from build123d import *

# Parameters (mm, degrees)
RECTANGLE130_AS_DRAWN_W                      = 25
RECTANGLE130_AS_DRAWN_H                      = 3
EXTRUDE152_DEPTH                             = 3
EXTRUDE152_ONTO_RECTANGLE130_ROLL_ANGLE      = -90
EXTRUDE152_ONTO_RECTANGLE130_PLACEMENT_ANGLE = 180
RECTANGLE128_AS_DRAWN_W                      = 25
RECTANGLE128_AS_DRAWN_H                      = 3
EXTRUDE153_DEPTH                             = 3
EXTRUDE153_ONTO_RECTANGLE128_ROLL_ANGLE      = -90
EXTRUDE153_ONTO_RECTANGLE128_PLACEMENT_ANGLE = 180
RECTANGLE132_AS_DRAWN_W                      = 3
RECTANGLE132_AS_DRAWN_H                      = 19.5
EXTRUDE166_DEPTH                             = 3
EXTRUDE166_ONTO_RECTANGLE132_ROLL_ANGLE      = -90
EXTRUDE166_ONTO_RECTANGLE132_PLACEMENT_ANGLE = 180
RECTANGLE127_AS_DRAWN_W                      = 25
RECTANGLE127_AS_DRAWN_H                      = 3
EXTRUDE147_DEPTH                             = 3
EXTRUDE147_ONTO_RECTANGLE127_ROLL_ANGLE      = -90
EXTRUDE147_ONTO_RECTANGLE127_PLACEMENT_ANGLE = 180
RECTANGLE129_AS_DRAWN_W                      = 25
RECTANGLE129_AS_DRAWN_H                      = 3
EXTRUDE149_DEPTH                             = 3
EXTRUDE149_ONTO_RECTANGLE129_ROLL_ANGLE      = -90
EXTRUDE149_ONTO_RECTANGLE129_PLACEMENT_ANGLE = 180
BOX045_W                                     = 100
BOX045_H                                     = 3
BOX045_DEPTH                                 = 45


with BuildPart() as extrude152:
    # Rectangle130 as drawn → Extrude152 (new)
    with BuildSketch(Plane.XY):
        with Locations((12.5, 1.5)):
            Rectangle(RECTANGLE130_AS_DRAWN_W, RECTANGLE130_AS_DRAWN_H)
    extrude(amount=-EXTRUDE152_DEPTH)


with BuildPart() as extrude152_1:
    # Extrude152 onto Rectangle130 roll: moved
    add(extrude152.part.rotate(Axis((0, 0, 0), (1, 0, 0)), EXTRUDE152_ONTO_RECTANGLE130_ROLL_ANGLE))


with BuildPart() as extrude152_2:
    # Extrude152 onto Rectangle130 placement: moved
    add(extrude152_1.part.moved(Location((39, -77, -70))).rotate(Axis((39, -77, -70), (0, 0, 1)), EXTRUDE152_ONTO_RECTANGLE130_PLACEMENT_ANGLE))


with BuildPart() as extrude152_3:
    # Extrude152 placement: moved
    add(extrude152_2.part.moved(Location((0, 0, -42))))


with BuildPart() as extrude153:
    # Rectangle128 as drawn → Extrude153 (new)
    with BuildSketch(Plane.XY):
        with Locations((12.5, 1.5)):
            Rectangle(RECTANGLE128_AS_DRAWN_W, RECTANGLE128_AS_DRAWN_H)
    extrude(amount=-EXTRUDE153_DEPTH)


with BuildPart() as extrude153_1:
    # Extrude153 onto Rectangle128 roll: moved
    add(extrude153.part.rotate(Axis((0, 0, 0), (1, 0, 0)), EXTRUDE153_ONTO_RECTANGLE128_ROLL_ANGLE))


with BuildPart() as extrude153_2:
    # Extrude153 onto Rectangle128 placement: moved
    add(extrude153_1.part.moved(Location((89, -77, -70))).rotate(Axis((89, -77, -70), (0, 0, 1)), EXTRUDE153_ONTO_RECTANGLE128_PLACEMENT_ANGLE))


with BuildPart() as extrude153_3:
    # Extrude153 placement: moved
    add(extrude153_2.part.moved(Location((0, 0, -42))))


with BuildPart() as extrude166:
    # Rectangle132 as drawn → Extrude166 (new)
    with BuildSketch(Plane.XY):
        with Locations((1.5, 9.75)):
            Rectangle(RECTANGLE132_AS_DRAWN_W, RECTANGLE132_AS_DRAWN_H)
    extrude(amount=-EXTRUDE166_DEPTH)


with BuildPart() as extrude166_1:
    # Extrude166 onto Rectangle132 roll: moved
    add(extrude166.part.rotate(Axis((0, 0, 0), (1, 0, 0)), EXTRUDE166_ONTO_RECTANGLE132_ROLL_ANGLE))


with BuildPart() as extrude166_2:
    # Extrude166 onto Rectangle132 placement: moved
    add(extrude166_1.part.moved(Location((114, -77, -92.5))).rotate(Axis((114, -77, -92.5), (0, 0, 1)), EXTRUDE166_ONTO_RECTANGLE132_PLACEMENT_ANGLE))


with BuildPart() as extrude147:
    # Rectangle127 as drawn → Extrude147 (new)
    with BuildSketch(Plane.XY):
        with Locations((12.5, 1.5)):
            Rectangle(RECTANGLE127_AS_DRAWN_W, RECTANGLE127_AS_DRAWN_H)
    extrude(amount=-EXTRUDE147_DEPTH)


with BuildPart() as extrude147_1:
    # Extrude147 onto Rectangle127 roll: moved
    add(extrude147.part.rotate(Axis((0, 0, 0), (1, 0, 0)), EXTRUDE147_ONTO_RECTANGLE127_ROLL_ANGLE))


with BuildPart() as extrude147_2:
    # Extrude147 onto Rectangle127 placement: moved
    add(extrude147_1.part.moved(Location((114, -77, -70))).rotate(Axis((114, -77, -70), (0, 0, 1)), EXTRUDE147_ONTO_RECTANGLE127_PLACEMENT_ANGLE))


with BuildPart() as fusion064026:
    # Rectangle129 as drawn → Extrude149 (new)
    with BuildSketch(Plane.XY):
        with Locations((12.5, 1.5)):
            Rectangle(RECTANGLE129_AS_DRAWN_W, RECTANGLE129_AS_DRAWN_H)
    extrude(amount=-EXTRUDE149_DEPTH)


with BuildPart() as fusion064026_1:
    # Extrude149 onto Rectangle129 roll: moved
    add(fusion064026.part.rotate(Axis((0, 0, 0), (1, 0, 0)), EXTRUDE149_ONTO_RECTANGLE129_ROLL_ANGLE))


with BuildPart() as fusion064026_2:
    # Extrude149 onto Rectangle129 placement: moved
    add(fusion064026_1.part.moved(Location((64, -77, -70))).rotate(Axis((64, -77, -70), (0, 0, 1)), EXTRUDE149_ONTO_RECTANGLE129_PLACEMENT_ANGLE))

    # Fusion064026: union Extrude152, Extrude153, Extrude166, Extrude147
    add(extrude152_3.part)
    add(extrude153_3.part)
    add(extrude166_2.part)
    add(extrude147_2.part)


with BuildPart() as fusion064026_3:
    # Fusion064026 placement: moved
    add(fusion064026_2.part.moved(Location((0, 152, 0))))


with BuildPart() as cut035015:
    # Box045 → Box045 (new body)
    with BuildSketch(Plane(origin=(14, 75, -115), x_dir=(1, 0, 0), z_dir=(0, 0, 1))):
        with Locations((50, 1.5)):
            Rectangle(BOX045_W, BOX045_H)
    extrude(amount=BOX045_DEPTH)

    # Cut035015: cut Fusion064026
    add(fusion064026_3.part, mode=Mode.SUBTRACT)


solid = cut035015.part
Geometry check sheet. Reference: the model listing, model coordinates, mm. A direction names the side the tool comes from. Give positions to 0.01 mm unless a question says otherwise; leave off trailing zeros. Order: outer loops, then holes, each group sorted by start corner. A loop starts at its lowest first (then second) coordinate and runs counter-clockwise, first axis right, second up. Notation, with made-up numbers: M 46.5,68 L 61.5,68 A22 cw 61.5,93 Z; hole C 87.25,44 d8. An arc over 180 degrees is marked long. Use a Markdown table: item, result.
Item 1: Section check C-C (z = -96). Record the cut outline in (x, y), and give its area (3 significant figures).
Answers follow:
| item | result |
|---|---|
| outline | M 14,75 L 111,75 L 111,78 L 14,78 Z |
| area | 291 mm2 |
Item 2: Depth check by flat-ended pin: P1, Ø1.5, axis at x = 49, y = 76.5, coming from the +Z side; P2, Ø1.5, axis at y = 77, z = -114, coming from the -X side; P3, Ø0.9, axis at y = 77, z = -100.5, coming from the +X side. Enter the tip coordinate at first touch or a pass-through.
Answers follow:
| item | result |
|---|---|
| P1 | stops at z = -73 |
| P2 | stops at x = 39 |
| P3 | stops at x = 111 |
Item 3: Material ranges on line 1 along X through (y, z) = (76.1, -112.5); line 2 along Z through (x, y) = (92, 76.4); line 3 along X through (y, z) = (75.8, -103), recorded low to high.
Answers follow:
| item | result |
|---|---|
| line 1 | x = 39 to 64, 89 to 114 |
| line 2 | z = -115 to -73 |
| line 3 | x = 14 to 111 |
Item 4: Tool access check on faces 5 (the flat face through (113, 76, -112)), 6 (the flat face through (39, 76, -113)), 7 (the flat face through (39, 76, -71)). Record the directions out of +Z, -Z, +X, -X, +Y, -Y that give a thin tool (end or side, any length) a straight path to the whole face; none if there is none.
Answers follow:
| item | result |
|---|---|
| face 5 | +X, +Y, -Y |
| face 6 | -Z, -X, +Y, -Y |
| face 7 | +Z, +Y, -Y |
Item 5: Draft check along X on faces 1 (the flat face through (14, 76, -91)), 2 (the flat face through (64, 76, -113)), 3 (the flat face through (89, 76, -113)), 4 (the flat face through (63, 75, -93)). Enter one of: +X half, -X half, draft (parallel to the pull), parting line (faces both ways), or undercut.
Answers follow:
| item | result |
|---|---|
| face 1 | -X half |
| face 2 | undercut |
| face 3 | undercut |
| face 4 | draft |
Item 6: Section check B-B (x = 46). Record the cut outline in (y, z).
Answers follow:
| item | result |
|---|---|
| outline | M 75,-115 L 78,-115 L 78,-73 L 75,-73 Z |
Item 7: Section check A-A (y = 76.85). Record the cut outline in (x, z), and give its area (3 significant figures).
Answers follow:
| item | result |
|---|---|
| outline | M 14,-112 L 39,-112 L 39,-115 L 64,-115 L 64,-112 L 89,-112 L 89,-115 L 114,-115 L 114,-112 L 111,-112 L 111,-92.5 L 114,-92.5 L 114,-73 L 89,-73 L 89,-70 L 64,-70 L 64,-73 L 39,-73 L 39,-70 L 14,-70 Z |
| area | 4,140 mm2 |
